from build123d import *

# Parameters (mm, degrees)
BOSS_EXTRUDE1_DEPTH = 2
SKETCH2_R           = 5
SKETCH2_R_2         = 2.5
SKETCH2_W           = 12
SKETCH2_H           = 30
CUT_EXTRUDE1_DEPTH  = 10


with BuildPart() as part:
    # Sketch1 → Boss-Extrude1 (new body)
    with BuildSketch(Plane(origin=(0, 0, 0), x_dir=(1, 0, 0), z_dir=(0, 1, 0))):
        Polygon((-130, 150), (-130, 130), (-150, 130), (-150, -130), (-130, -130), (-130, -150), (130, -150), (130, -130), (150, -130), (150, 130), (130, 130), (130, 150), align=None)
    extrude(amount=BOSS_EXTRUDE1_DEPTH)

    # Sketch2 → Cut-Extrude1 (cut)
    with BuildSketch(Plane(origin=(0, 2, 0), x_dir=(1, 0, 0), z_dir=(0, 1, 0))):
        with Locations((100, 100)):
            Circle(SKETCH2_R)
        with Locations((56.45, -2.85)):
            Circle(SKETCH2_R_2)
        with Locations((40.45, -2.85)):
            Circle(SKETCH2_R_2)
        with Locations((40.45, -36.85)):
            Circle(SKETCH2_R_2)
        with Locations((56.45, -36.85)):
            Circle(SKETCH2_R_2)
        with Locations((0, -30)):
            Rectangle(SKETCH2_W, SKETCH2_H)
        with Locations((0, 80)):
            Rectangle(SKETCH2_W, SKETCH2_H)
    extrude(amount=-CUT_EXTRUDE1_DEPTH, mode=Mode.SUBTRACT)


solid = part.part
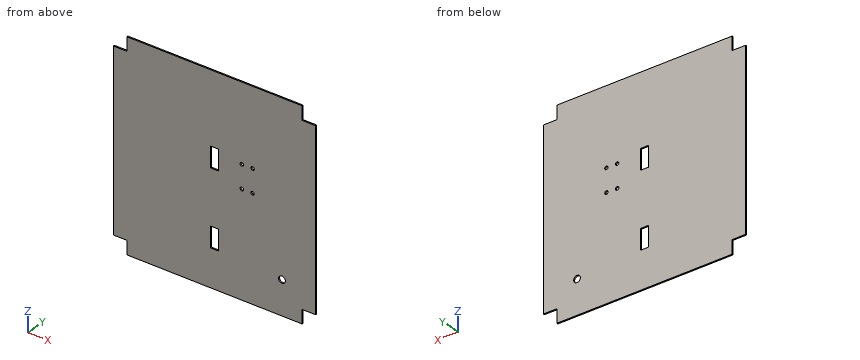
Work out the finished part from the listing and answer in its coordinate system (mm). Coordinates: 2 decimals unless noted, no trailing zeros. Loops run counter-clockwise (first coordinate to the right, second up) from the corner with the lowest first, then second, coordinate; pieces in that order, holes last. Notation, with made-up numbers: (30.25, -1) -> (76.25, -1) arc R18 ccw to (76.25, 28) -> close; hole circle Ø7 at (43, 49). An arc over 180 degrees is marked (long way). Answer as CSV lines item,"result".
1) The part is cut by section A-A (z = 19.5). Give the vertices of the cut face in (x, y), and give its area (3 significant figures).
A:
outline,"(-150, 0) -> (-6, 0) -> (-6, 2) -> (-150, 2) -> close; (6, 0) -> (150, 0) -> (150, 2) -> (6, 2) -> close"
area,"576 mm²"
2) The part is cut by section B-B (y = 1.4). Give the vertices of the cut face in (x, z), and give its area (3 significant figures).
A:
outline,"(-150, -130) -> (-130, -130) -> (-130, -150) -> (130, -150) -> (130, -130) -> (150, -130) -> (150, 130) -> (130, 130) -> (130, 150) -> (-130, 150) -> (-130, 130) -> (-150, 130) -> close; hole (-6, -95) -> (6, -95) -> (6, -65) -> (-6, -65) -> close; hole (-6, 15) -> (6, 15) -> (6, 45) -> (-6, 45) -> close; hole circle Ø5 at (40.45, 2.85); hole circle Ø5 at (40.45, 36.85); hole circle Ø5 at (56.45, 2.85); hole circle Ø5 at (56.45, 36.85); hole circle Ø10 at (100, -100)"
area,"87,500 mm²"
3) The part is cut by section C-C (z = -100). Give the vertices of the cut face in (x, y), and give its area (3 significant figures).
A:
outline,"(-150, 0) -> (95, 0) -> (95, 2) -> (-150, 2) -> close; (105, 0) -> (150, 0) -> (150, 2) -> (105, 2) -> close"
area,"580 mm²"
4) A flat-ended cylindrical pin translates along its axis: pin 1 (0.6 mm diameter, centred on y = 1.5, z = -137.5, fed in from -X). Find the tip coordinate at first contact, or state that the pin passes through.
A:
pin 1,"stops at x = -130"
5) Straight lines are drawn through the part: probe 1 along X at (y, z) = (0.85, 36.85); probe 2 along Z at (x, y) = (56.45, 1.5); probe 3 along X at (y, z) = (1, 2.85). For each, find the intervals that lie inside material, in ascending order.
A:
probe 1,"x = -150 to -6, 6 to 37.95, 42.95 to 53.95, 58.95 to 150"
probe 2,"z = -150 to 0.35, 5.35 to 34.35, 39.35 to 150"
probe 3,"x = -150 to 37.95, 42.95 to 53.95, 58.95 to 150"
